Read the model definition and answer for the solid it produces. Units are mm, in the model's axes. A direction names the side the tool comes from. Coordinates: 2 decimals unless noted, no trailing zeros. Write each loop counter-clockwise with the first axis right and the second up, starting at its lowest first coordinate (ties: lowest second). Pieces come first, ordered by that corner, then holes. Notation, with made-up numbers: (63.5, 11) -> (115.5, 11) arc R35 cw to (115.5, 43) -> close; hole circle Ø3 at (87.25, -5). An arc over 180 degrees is marked (long way). Answer as a JSON object with one key per item and string values. Group by question number.
(1) Find section D-D (x = 75). Give the vertices of the cut face in (y, z).
(2) Find section B-B (x = 25). Give the vertices of the cut face in (y, z).
(3) Which of the six approach directions +Z, -Z, +X, -X, +Y, -Y give full straight-line access (tool end or side, diameter ignored) to faces 5 (the face through (69.5, -30.1, 14.9)), 6 (the face through (75, -25, 20)), 7 (the face through (10, -25, 20))?
(4) Find section C-C (y = -28). Give the vertices of the cut face in (x, z).
(5) For a pull along X with two mould halves and no side action, classify faces 1 (the face through (100, -25, 5)), 2 (the face through (31, -19, 50)), 3 (the face through (19.5, -19.9, 45.1)), 4 (the face through (81, -19, 10)) as +X half, -X half, draft (parallel to the pull), parting line (faces both ways), or undercut.
(6) Find section A-A (z = 4.5). Give the vertices of the cut face in (x, y), then the cut area to 3 significant figures.
(7) Straight lines are drawn through the part: L1, parallel to X at y = -41.5, z = 15; L2, parallel to Y at x = 25, z = 43; L3, parallel to X at y = -2.5, z = 4.5. For each, find the intervals that lie inside material, in ascending order.
(8) Flat-ended cylindrical pins translate along their axes: P1, Ø9, axis at x = 25, y = -25, coming from the +Z side; P2, Ø15, axis at x = 73.5, y = -28.5, coming from the +Z side; P3, Ø9, axis at x = 21, y = -29.5, coming from the -Z side; P4, Ø6, axis at y = -7, z = 20, coming from the +X side. Find the tip coordinate at first contact, or state that the pin passes through.
from build123d import *

# Parameters (mm, degrees)
F1_DEPTH = 50
F2_W     = 30
F2_H     = 40
F3_DEPTH = 50.001
F4_R     = 7.5
F5_DEPTH = 50.001
F6_R     = 7.5
F7_DEPTH = 20


with BuildPart() as f1:
    # F0 (on Front) → F1 (new body)
    with BuildSketch(Plane.XZ):
        Polygon((0, 50), (0, 0), (100, 0), (100, 10), (50, 10), (50, 50), align=None)
    extrude(amount=F1_DEPTH)

    # F2 (on face) → F3 (cut, through all)
    with BuildSketch(Plane.XZ.offset(50)):
        with Locations((25, 20)):
            Rectangle(F2_W, F2_H)
    extrude(amount=-F3_DEPTH, mode=Mode.SUBTRACT)

    # F4 (on face) → F5 (cut, through all)
    with BuildSketch(Plane.XY.offset(50)):
        with Locations((25, -25.001487)):
            Circle(F4_R)
    extrude(amount=-F5_DEPTH, mode=Mode.SUBTRACT)

    # F6 (on face) → F7 (join)
    with BuildSketch(Plane(origin=(0, 0, 0), x_dir=(1, 0, 0), z_dir=(0, 0, -1))):
        with Locations((75, 25)):
            Circle(F6_R)
    extrude(amount=-F7_DEPTH)


solid = f1.part
Results below:
{
 "1": {"outline": "(-50, 0) -> (0, 0) -> (0, 10) -> (-17.5, 10) -> (-17.5, 20) -> (-32.5, 20) -> (-32.5, 10) -> (-50, 10) -> close"},
 "2": {"outline": "(-50, 40) -> (-32.5, 40) -> (-32.5, 50) -> (-50, 50) -> close; (-17.5, 40) -> (0, 40) -> (0, 50) -> (-17.5, 50) -> close"},
 "3": {"face 5": "+Z", "face 6": "+Z, +X, +Y, -Y", "face 7": "-Z, +Y, -Y"},
 "4": {"outline": "(0, 0) -> (10, 0) -> (10, 40) -> (18.13, 40) -> (18.13, 50) -> (0, 50) -> close; (31.87, 40) -> (40, 40) -> (40, 0) -> (100, 0) -> (100, 10) -> (81.87, 10) -> (81.87, 20) -> (68.13, 20) -> (68.13, 10) -> (50, 10) -> (50, 50) -> (31.87, 50) -> close"},
 "5": {"face 1": "+X half", "face 2": "draft", "face 3": "undercut", "face 4": "undercut"},
 "6": {"outline": "(0, -50) -> (10, -50) -> (10, 0) -> (0, 0) -> close; (40, -50) -> (100, -50) -> (100, 0) -> (40, 0) -> close", "area": "3,500 mm2"},
 "7": {"L1": "x = 0 to 10, 40 to 50", "L2": "y = -50 to -32.5, -17.5 to 0", "L3": "x = 0 to 10, 40 to 100"},
 "8": {"P1": "passes through", "P2": "stops at z = 20", "P3": "stops at z = 40", "P4": "stops at x = 50"}
}
